Build history of the part. All positions in model axes, mm. Face numbers are marked on the shaded views. A direction names the side the tool comes from. Coordinates: 2 decimals unless noted, no trailing zeros. Write each loop counter-clockwise with the first axis right and the second up, starting at its lowest first coordinate (ties: lowest second). Pieces come first, ordered by that corner, then holes.
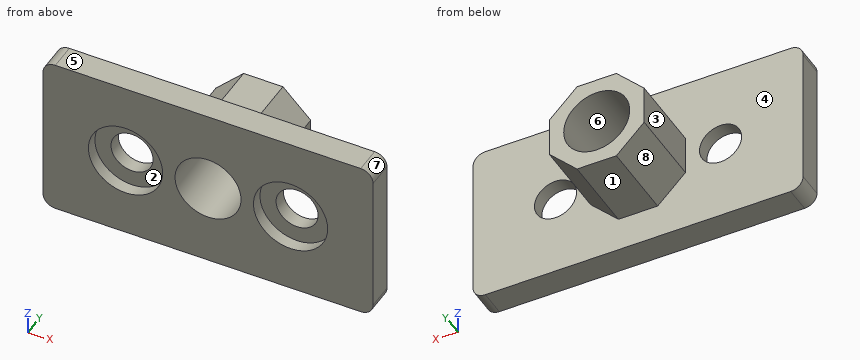
```python
from build123d import *

# Parameters (mm, degrees)
SKETCH1_W           = 40
SKETCH1_H           = 3.2
BOSS_EXTRUDE1_DEPTH = 20
SKETCH3_R           = 2.55
CUT_EXTRUDE2_DEPTH  = 4.2
SKETCH5_R           = 4.5
CUT_EXTRUDE4_DEPTH  = 1.5
BOSS_EXTRUDE2_DEPTH = 9.5
SKETCH7_R           = 4
CUT_EXTRUDE5_DEPTH  = 13.7
FILLET1_R           = 1.5


with BuildPart() as part:
    # Sketch1 → Boss-Extrude1 (new body)
    with BuildSketch(Plane.XY):
        Rectangle(SKETCH1_W, SKETCH1_H)
    extrude(amount=BOSS_EXTRUDE1_DEPTH)

    # Sketch3 → Cut-Extrude2 (cut, through all)
    with BuildSketch(Plane(origin=(0, 1.6, 0), x_dir=(1, 0, 0), z_dir=(0, 1, 0))):
        with Locations((-10, -10)):
            Circle(SKETCH3_R)
        with Locations((10, -10)):
            Circle(SKETCH3_R)
    extrude(amount=-CUT_EXTRUDE2_DEPTH, mode=Mode.SUBTRACT)

    # Sketch5 → Cut-Extrude4 (cut)
    with BuildSketch(Plane.XZ.offset(1.6)):
        with Locations((10, 10)):
            Circle(SKETCH5_R)
        with Locations((-10, 10)):
            Circle(SKETCH5_R)
    extrude(amount=-CUT_EXTRUDE4_DEPTH, mode=Mode.SUBTRACT)

    # Sketch6 → Boss-Extrude2 (add)
    with BuildSketch(Plane(origin=(0, 1.6, 0), x_dir=(1, 0, 0), z_dir=(0, 1, 0))):
        Polygon((-2.381727984, -4.25), (-5.75, -7.618272016), (-5.75, -12.381727984), (-2.381727984, -15.75), (2.381727984, -15.75), (5.75, -12.381727984), (5.75, -7.618272016), (2.381727984, -4.25), align=None)
    extrude(amount=BOSS_EXTRUDE2_DEPTH)

    # Sketch7 → Cut-Extrude5 (cut, through all)
    with BuildSketch(Plane(origin=(0, 11.1, 0), x_dir=(1, 0, 0), z_dir=(0, 1, 0))):
        with Locations((0, -10)):
            Circle(SKETCH7_R)
    extrude(amount=-CUT_EXTRUDE5_DEPTH, mode=Mode.SUBTRACT)

    # Fillet1
    fillet1_edges = [part.edges().sort_by_distance(p)[0] for p in [
        (20, 0, 20),
        (-20, 0, 20),
        (20, 0, 0),
        (-20, 0, 0),
    ]]
    fillet(fillet1_edges, radius=FILLET1_R)


solid = part.part
```
1. Saw through at C-C on x = -10. List the corners of the cut face in (y, z).
Computed values:
outline: (-1.6, 0) - (1.6, 0) - (1.6, 7.45) - (-0.1, 7.45) - (-0.1, 5.5) - (-1.6, 5.5) - close; (-1.6, 14.5) - (-0.1, 14.5) - (-0.1, 12.55) - (1.6, 12.55) - (1.6, 20) - (-1.6, 20) - close
2. Probe line 1 along X through (y, z) = (0.5, 10); line 2 along Z through (x, y) = (10, 1.3); line 3 along Z through (x, y) = (10, -1). List the from-to ranges inside material, lowest first.
Computed values:
line 1: x = -20 to -12.55, -7.45 to -4, 4 to 7.45, 12.55 to 20
line 2: z = 0 to 7.45, 12.55 to 20
line 3: z = 0 to 5.5, 14.5 to 20
3. Saw through at A-A on x = 0. List the corners of the cut face in (y, z), plus the area to 4 significant figures.
Computed values:
outline: (-1.6, 0) - (1.6, 0) - (1.6, 4.25) - (11.1, 4.25) - (11.1, 6) - (-1.6, 6) - close; (-1.6, 14) - (11.1, 14) - (11.1, 15.75) - (1.6, 15.75) - (1.6, 20) - (-1.6, 20) - close
area: 71.65 mm2
4. 3-axis set-ups, long thin cutter, end or side, ignore diameter. For the marked faces 1, 2, 3 and 4: which of +Z, -Z, +X, -X, +Y, -Y reach the whole face in a straight line?
Computed values:
face 1: -Z, +X, -X, +Y
face 2: -Y
face 3: +Z, -Z, -X, +Y
face 4: +Y
5. Flat gauge pins, fed straight in: pin 1 (2.5 mm diameter, centred on x = 11, z = 9.5, fed in from -Y); pin 2 (6.5 mm diameter, centred on x = 10, z = 10, fed in from -Y); pin 3 (1.4 mm diameter, centred on y = 5.5, z = 10.5, fed in from -X); pin 4 (1.4 mm diameter, centred on y = 5.5, z = 10.5, fed in from +X). Where does each tip first touch, or does it go through?
Computed values:
pin 1: passes through
pin 2: stops at y = -0.1
pin 3: stops at x = -5.75
pin 4: stops at x = 5.75
6. Mould opens along X. For the marked faces 5, 6, 7 and 8 say: +X half, -X half, draft (parallel to the pull), parting line (faces both ways), or undercut.
Computed values:
face 5: draft
face 6: undercut
face 7: +X half
face 8: -X half
7. Saw through at D-D on z = 2. List the corners of the cut face in (x, y), plus the area to 3 significant figures.
Computed values:
outline: (-20, -1.6) - (20, -1.6) - (20, 1.6) - (-20, 1.6) - close
area: 128 mm2
8. Saw through at B-B on y = 4. List the corners of the cut face in (x, z).
Computed values:
outline: (-5.75, 7.62) - (-2.38, 4.25) - (2.38, 4.25) - (5.75, 7.62) - (5.75, 12.38) - (2.38, 15.75) - (-2.38, 15.75) - (-5.75, 12.38) - close; hole circle Ø8 at (0, 10)
